Work out the finished part from the listing and answer in its coordinate system (mm). Give positions to 0.01 mm unless a question says otherwise; leave off trailing zeros. Loops run counter-clockwise (first coordinate to the right, second up) from the corner with the lowest first, then second, coordinate; pieces in that order, holes last.
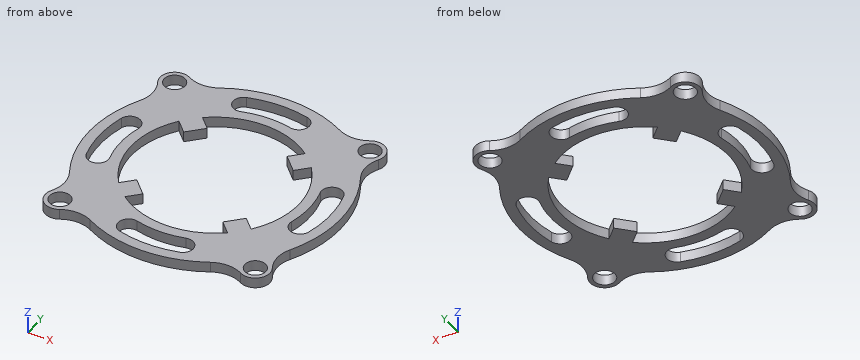
```python
from build123d import *

# Parameters (mm, degrees)
ESBO_O1_R                = 120
ESBO_O1_R_2              = 80
RESSALTO_EXTRUS_O1_DEPTH = 10
CORTE_EXTRUS_O1_DEPTH    = 10
ESBO_O3_R                = 14
ESBO_O3_R_2              = 10
RESSALTO_EXTRUS_O2_DEPTH = 10
FILETE1_R                = 30
RESSALTO_EXTRUS_O3_START = -10
RESSALTO_EXTRUS_O3_DEPTH = 10


with BuildPart() as part:
    # Esboço1 → Ressalto-extrusão1 (new body)
    with BuildSketch(Plane.XY):
        Circle(ESBO_O1_R)
        Circle(ESBO_O1_R_2, mode=Mode.SUBTRACT)
    extrude(amount=RESSALTO_EXTRUS_O1_DEPTH)

    # Esboço2 → Corte-extrusão1 (cut)
    with BuildSketch(Plane.XY.offset(10)):
        with BuildLine():
            ThreePointArc((25.245684703, 107.063791283), (-3.324689368, 109.949745068), (-31.668491353, 105.342805428))
            ThreePointArc((-31.668491353, 105.342805428), (-38.366156269, 92.887232993), (-25.910583834, 86.189568077))
            ThreePointArc((-25.910583834, 86.189568077), (-2.720200392, 89.958882329), (20.655560211, 87.597647413))
            ThreePointArc((20.655560211, 87.597647413), (32.683694392, 95.035657102), (25.245684703, 107.063791283))
        make_face()
        with BuildLine():
            ThreePointArc((106.251840892, -28.470094961), (110, 0), (106.251840892, 28.470094961))
            ThreePointArc((106.251840892, 28.470094961), (94.004392178, 35.541162773), (86.933324366, 23.293714059))
            ThreePointArc((86.933324366, 23.293714059), (90, 0), (86.933324366, -23.293714059))
            ThreePointArc((86.933324366, -23.293714059), (94.004392178, -35.541162773), (106.251840892, -28.470094961))
        make_face()
        with BuildLine():
            ThreePointArc((-28.470094961, -106.251840892), (0, -110), (28.470094961, -106.251840892))
            ThreePointArc((28.470094961, -106.251840892), (35.541162773, -94.004392178), (23.293714059, -86.933324366))
            ThreePointArc((23.293714059, -86.933324366), (0, -90), (-23.293714059, -86.933324366))
            ThreePointArc((-23.293714059, -86.933324366), (-35.541162773, -94.004392178), (-28.470094961, -106.251840892))
        make_face()
        with BuildLine():
            ThreePointArc((-106.251840892, 28.470094961), (-110, 0), (-106.251840892, -28.470094961))
            ThreePointArc((-106.251840892, -28.470094961), (-94.004392178, -35.541162773), (-86.933324366, -23.293714059))
            ThreePointArc((-86.933324366, -23.293714059), (-90, 0), (-86.933324366, 23.293714059))
            ThreePointArc((-86.933324366, 23.293714059), (-94.004392178, 35.541162773), (-106.251840892, 28.470094961))
        make_face()
    extrude(amount=-CORTE_EXTRUS_O1_DEPTH, mode=Mode.SUBTRACT)

    # Esboço3 → Ressalto-extrusão2 (add)
    # profile 1 of 4: a face of its own
    with BuildSketch(Plane.XY.offset(10)):
        with Locations((93.338095117, 93.338095117)):
            Circle(ESBO_O3_R)
        with Locations((93.338095117, 93.338095117)):
            Circle(ESBO_O3_R_2, mode=Mode.SUBTRACT)
    # profile 2 of 4: a face of its own
    with BuildSketch(Plane.XY.offset(10)):
        with Locations((93.338095117, -93.338095117)):
            Circle(ESBO_O3_R)
        with Locations((93.338095117, -93.338095117)):
            Circle(ESBO_O3_R_2, mode=Mode.SUBTRACT)
    # profile 3 of 4: a face of its own
    with BuildSketch(Plane.XY.offset(10)):
        with Locations((-93.338095117, -93.338095117)):
            Circle(ESBO_O3_R)
        with Locations((-93.338095117, -93.338095117)):
            Circle(ESBO_O3_R_2, mode=Mode.SUBTRACT)
    # profile 4 of 4: a face of its own
    with BuildSketch(Plane.XY.offset(10)):
        with Locations((-93.338095117, 93.338095117)):
            Circle(ESBO_O3_R)
        with Locations((-93.338095117, 93.338095117)):
            Circle(ESBO_O3_R_2, mode=Mode.SUBTRACT)
    extrude(amount=-RESSALTO_EXTRUS_O2_DEPTH)

    # Filete1
    filete1_edges = [part.edges().sort_by_distance(p)[0] for p in [
        (-89.573264047, -79.853806221, 5),
        (-79.853806221, -89.573264047, 5),
        (-79.853806221, 89.573264047, 5),
        (-89.573264047, 79.853806221, 5),
        (79.853806221, 89.573264047, 5),
        (89.573264047, 79.853806221, 5),
        (89.573264047, -79.853806221, 5),
        (79.853806221, -89.573264047, 5),
    ]]
    fillet(filete1_edges, radius=FILETE1_R)

    # Esboço4 → Ressalto-extrusão3 (add)
    with BuildSketch(Plane.XY.offset(10).offset(RESSALTO_EXTRUS_O3_START)):
        with BuildLine():
            Line((52.325901808, -38.183766184), (38.183766184, -52.325901808))
            Line((38.183766184, -52.325901808), (49.05379299, -63.195928613))
            ThreePointArc((49.05379299, -63.195928613), (56.568542495, -56.568542495), (63.195928613, -49.05379299))
            Line((63.195928613, -49.05379299), (52.325901808, -38.183766184))
        make_face()
        with BuildLine():
            Line((-38.183766184, -52.325901808), (-52.325901808, -38.183766184))
            Line((-52.325901808, -38.183766184), (-63.195928613, -49.05379299))
            ThreePointArc((-63.195928613, -49.05379299), (-56.568542495, -56.568542495), (-49.05379299, -63.195928613))
            Line((-49.05379299, -63.195928613), (-38.183766184, -52.325901808))
        make_face()
        with BuildLine():
            Line((38.183766184, 52.325901808), (52.325901808, 38.183766184))
            Line((52.325901808, 38.183766184), (63.195928613, 49.05379299))
            ThreePointArc((63.195928613, 49.05379299), (56.568542495, 56.568542495), (49.05379299, 63.195928613))
            Line((49.05379299, 63.195928613), (38.183766184, 52.325901808))
        make_face()
        with BuildLine():
            Line((-52.325901808, 38.183766184), (-38.183766184, 52.325901808))
            Line((-38.183766184, 52.325901808), (-49.05379299, 63.195928613))
            ThreePointArc((-49.05379299, 63.195928613), (-56.568542495, 56.568542495), (-63.195928613, 49.05379299))
            Line((-63.195928613, 49.05379299), (-52.325901808, 38.183766184))
        make_face()
    extrude(amount=RESSALTO_EXTRUS_O3_DEPTH)


solid = part.part
```
Q1. Given pin 1 (5 mm diameter, centred on x = 53, z = 3.5, fed in from +Y); pin 2 (2 mm diameter, centred on x = -38.5, z = 7.5, fed in from +Y); pin 3 (1.5 mm diameter, centred on x = 90, z = 5, fed in from -Y), each flat-ended and moving along its own axis, determine where each tip first touches the part or whether it passes through.
Q2. Section C-C on z = 2.75 is taken. State how many separate pieces and enclosed holes the cut face has, plus the area to 3 significant figures.
Q3. Section A-A on y = -20 is taken. Give the vertices of the cut face in (x, z), plus the area to 3 significant figures.
Q4. Consider line 1 along X through (y, z) = (1, 9.75); line 2 along Y through (x, z) = (20.5, 1.25). Determine where each line is inside the solid, lowest interval first.
Q5. Section B-B on y = 46 is taken. Give the vertices of the cut face in (x, z).
Check result:
1. pin 1: stops at y = 108.86
1. pin 2: stops at y = 113.99
1. pin 3: stops at y = -107.1
2. separate pieces: 1
2. enclosed holes: 9
2. area: 22,900 mm2
3. outline: (-118.32, 0) - (-108.17, 0) - (-108.17, 10) - (-118.32, 10) - close; (-87.75, 0) - (-77.46, 0) - (-77.46, 10) - (-87.75, 10) - close; (77.46, 0) - (87.75, 0) - (87.75, 10) - (77.46, 10) - close; (108.17, 0) - (118.32, 0) - (118.32, 10) - (108.17, 10) - close
3. area: 409 mm2
4. line 1: x = -120 to -110, -89.99 to -79.99, 79.99 to 89.99, 110 to 120
4. line 2: y = -118.24 to -108.07, -87.63 to -77.33, 77.33 to 87.63, 108.07 to 118.24
5. outline: (-110.83, 0) - (-65.45, 0) - (-65.45, 10) - (-110.83, 10) - close; (-60.14, 0) - (-44.51, 0) - (-44.51, 10) - (-60.14, 10) - close; (44.51, 0) - (60.14, 0) - (60.14, 10) - (44.51, 10) - close; (65.45, 0) - (110.83, 0) - (110.83, 10) - (65.45, 10) - close
